from build123d import *

# Parameters (mm, degrees)
F0_R     = 2.6
F1_DEPTH = 6.5024


with BuildPart() as f1:
    # F0 (on Top) → F1 (new body)
    with BuildSketch(Plane.XY):
        with BuildLine():
            Line((-103, 75), (-120, 75))
            Line((-120, 75), (-170, 25))
            Line((-170, 25), (-170, 3))
            ThreePointArc((-170, 3), (-169.12132, 0.87868), (-167, 0))
            Line((-167, 0), (0, 0))
            Line((0, 0), (167, 0))
            ThreePointArc((167, 0), (169.12132, 0.87868), (170, 3))
            Line((170, 3), (170, 25))
            Line((170, 25), (120, 75))
            Line((120, 75), (103, 75))
            ThreePointArc((103, 75), (100.87868, 75.87868), (100, 78))
            Line((100, 78), (100, 117))
            ThreePointArc((100, 117), (99.12132, 119.12132), (97, 120))
            Line((97, 120), (0, 120))
            Line((0, 120), (-97, 120))
            ThreePointArc((-97, 120), (-99.12132, 119.12132), (-100, 117))
            Line((-100, 117), (-100, 78))
            ThreePointArc((-100, 78), (-100.87868, 75.87868), (-103, 75))
        make_face()
        with Locations((-80, 81.9)):
            Circle(F0_R, mode=Mode.SUBTRACT)
        with Locations((-80, 107.3)):
            Circle(F0_R, mode=Mode.SUBTRACT)
        with Locations((80, 81.9)):
            Circle(F0_R, mode=Mode.SUBTRACT)
        with Locations((80, 107.3)):
            Circle(F0_R, mode=Mode.SUBTRACT)
    extrude(amount=F1_DEPTH)


solid = f1.part
Part model, mm, in its own coordinate system. A direction names the side the tool comes from. Round coordinates to 2 decimals unless told otherwise and drop trailing zeros. Write each loop counter-clockwise with the first axis right and the second up, starting at its lowest first coordinate (ties: lowest second). Pieces come first, ordered by that corner, then holes. Notation, with made-up numbers: (28.5, 12) - (87.5, 12) arc R10 cw to (87.5, 28) - close; hole circle Ø4 at (-29, 24.25). An arc over 180 degrees is marked (long way). Use CSV: the item, a comma, the result in double quotes.
Item 1: Flat gauge pins, fed straight in: P1, Ø3.5, axis at x = -112, z = 4, coming from the +Y side; P2, Ø2, axis at y = 100, z = 3.5, coming from the -X side; P3, Ø10, axis at x = -109.5, y = 99.5, coming from the +Z side; P4, Ø2, axis at y = 103.5, z = 2, coming from the +X side. Where does each tip first touch, or does it go through?
Results list:
P1,"stops at y = 75"
P2,"stops at x = -100"
P3,"passes through"
P4,"stops at x = 100"
Item 2: Slice it at A-A, the plane z = 3. Write the cut outline in (x, y), then the cut area to 3 significant figures.
Results list:
outline,"(-170, 3) arc R3 ccw to (-167, 0) - (167, 0) arc R3 ccw to (170, 3) - (170, 25) - (120, 75) - (103, 75) arc R3 cw to (100, 78) - (100, 117) arc R3 ccw to (97, 120) - (-97, 120) arc R3 ccw to (-100, 117) - (-100, 78) arc R3 cw to (-103, 75) - (-120, 75) - (-170, 25) - close; hole circle Ø5.2 at (-80, 81.9); hole circle Ø5.2 at (-80, 107.3); hole circle Ø5.2 at (80, 81.9); hole circle Ø5.2 at (80, 107.3)"
area,"31,900 mm²"
Item 3: Slice it at B-B, the plane y = 37. Write the cut outline in (x, z), then the cut area to 3 significant figures.
Results list:
outline,"(-158, 0) - (158, 0) - (158, 6.5) - (-158, 6.5) - close"
area,"2,050 mm²"
Item 4: Tool access for faces 1 (the flat face through (-2, 48, 0)), 2 (the flat face through (112, 75, 3)), 3 (the flat face through (-111, 75, 3)): list every direction of +Z, -Z, +X, -X, +Y, -Y with a clear straight run to the whole face (end or side of a thin tool).
Results list:
face 1,"-Z, +X, -X, +Y, -Y"
face 2,"+Z, -Z, +X, +Y"
face 3,"+Z, -Z, -X, +Y"
Item 5: Wall check: L1, parallel to Y at x = 80, z = 4.5; L2, parallel to Y at x = 108, z = 3.75; L3, parallel to X at y = 89, z = 3.5. Give the ranges that are in metal, low to high.
Results list:
L1,"y = 0 to 79.3, 84.5 to 104.7, 109.9 to 120"
L2,"y = 0 to 75"
L3,"x = -100 to 100"
Item 6: Slice it at C-C, the plane x = 141. Write the cut outline in (y, z).
Results list:
outline,"(0, 0) - (54, 0) - (54, 6.5) - (0, 6.5) - close"
